Autodesk Inventor part; units mm, degrees
ref_plane "Work Plane1" through (0, 5, 0) normal (0, 1, 0) x (-1, 0, 0)
ref_plane "YZ Plane" through (0, 0, 0) normal (1, 0, 0) x (0, 1, 0)
ref_plane "XY Plane" through (0, 0, 0) normal (0, 0, 1) x (1, 0, 0)
sketch "Sketch5" plane through (0, 0, 0) normal (1, 0, 0) x (0, 1, 0)
  line L0 (0, 0) -> (5, 0)
  line L1 (5, 0) -> (5, -1.5)
  line L2 (5, -1.5) -> (3.55, -1.5)
  line L3 (3.55, -1.5) -> (3.55, -2.4)
  line L4 (3.55, -2.4) -> (5, -2.4)
  line L5 (5, -2.4) -> (5, -23.9)
  line L6 (5, -23.9) -> (3.55, -23.9)
  line L7 (3.55, -23.9) -> (3.55, -24.8)
  line L8 (3.55, -24.8) -> (5, -24.8)
  line L9 (5, -24.8) -> (5, -50)
  line L10 (5, -50) -> (0, -50)
  line L11 (0, -50) -> (0, 0)
  dimension "d14" = 0.9
  dimension "d15" = 1.5
  dimension "d16" = 0.9
  dimension "d17" = 50
  dimension "d18" = 10
  dimension "d19" = 7.1
  dimension "d28" = 23.3
revolve "Revolution2" add sketch "Sketch5" angle 360 about axis through (0, 0, -50) along (0, 0, 1)
ref_plane "Work Plane1" through (0, 5, 0) normal (0, 1, 0) x (-1, 0, 0)
sketch "Sketch6" plane through (0, 5, 0) normal (0, 1, 0) x (-1, 0, 0)
  line L0 (0, -5.5) -> (0, -9.5) construction
  line L1 (-2, -5.5) -> (-2, -9.5)
  line L2 (2, -9.5) -> (2, -5.5)
  arc A0 (2, -5.5) -> (-2, -5.5) centre (0, -5.5) ccw
  arc A1 (-2, -9.5) -> (2, -9.5) centre (0, -9.5) ccw
  line L3 (5, -1.5) -> (-5, -1.5)
  point P0 (0, 0)
  point P1 (0, -7.5)
  point P2 (0, -3.5)
  point P3 (0, -11.5)
  dimension "d22" = 4
  dimension "d23" = 8
  dimension "d24" = 2
extrude "Extrusion4" cut sketch "Sketch6" against normal blind 2.3
properties part number "gearbox_shaft2" material "Steel"
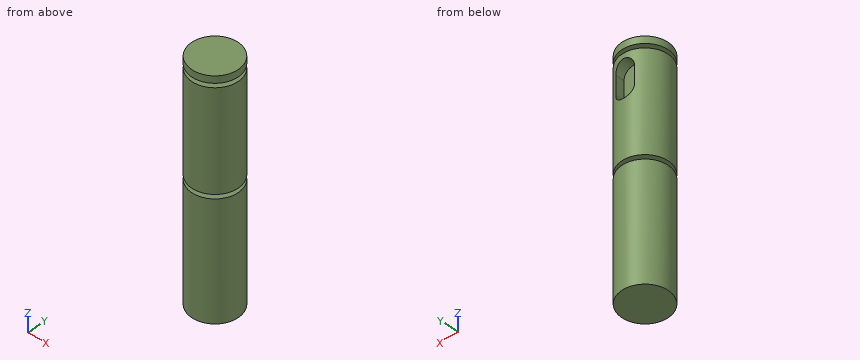
Can you work these out from the model? Positions are in its coordinate system, mm. Give positions to 0.01 mm unless a question says otherwise; leave off trailing zeros. Loops run counter-clockwise (first coordinate to the right, second up) from the corner with the lowest first, then second, coordinate; pieces in that order, holes last. Notation, with made-up numbers: M 51.25,64.25 L 90.25,64.25 A34 ccw 90.25,97.25 Z; hole C 77.25,-7.5 d6. An arc over 180 degrees is marked long. Use CSV: the item, a comma, the result in double quotes. Start each with the question number.
1. Imagine slicing it at A-A, the plane x = -4.25. Write out the boundary of the cut face in (y, z).
2. Imagine slicing it at D-D, the plane z = -41.5. Write out the boundary of the cut face in (x, y), plus the area to 3 significant figures.
3. If I drill on L1, parallel to Z at x = -1.75, y = -3.5; L2, parallel to Y at x = 3.75, z = -34.5; L3, parallel to Y at x = 1, z = -21, over which ranges is the centre line in solid material (lowest first)?
4. Imagine slicing it at B-B, the plane x = -0.5. Write out the boundary of the cut face in (y, z), plus the area to 3 significant figures.
5. Imagine slicing it at C-C, the plane y = -1.5. Write out the boundary of the cut face in (x, z), plus the area to 3 significant figures.
6. For P1, Ø4.5, axis at x = 0.5, z = -6, coming from the +Y side; P2, Ø1, axis at y = -3.5, z = -33, coming from the -X side; P3, Ø0.6, axis at y = 4, z = -8, coming from the +X side, each with a flat end and sliding along its axis, tell me the tip position at first contact or that it passes through.
Response values:
1,outline,"M -2.63,-50 L 2.63,-50 L 2.63,-24.8 L -2.63,-24.8 Z; M -2.63,-23.9 L 2.63,-23.9 L 2.63,-2.4 L -2.63,-2.4 Z; M -2.63,-1.5 L 2.63,-1.5 L 2.63,0 L -2.63,0 Z"
2,outline,"C 0,0 d10"
2,area,"78.5 mm^2"
3,L1,"-50 to -24.8, -23.9 to -2.4, -1.5 to 0"
3,L2,"-3.31 to 3.31"
3,L3,"-4.9 to 4.9"
4,outline,"M -4.97,-50 L 4.97,-50 L 4.97,-24.8 L 3.51,-24.8 L 3.51,-23.9 L 4.97,-23.9 L 4.97,-11.44 L 2.7,-11.44 L 2.7,-3.56 L 4.97,-3.56 L 4.97,-2.4 L 3.51,-2.4 L 3.51,-1.5 L 4.97,-1.5 L 4.97,0 L -4.97,0 L -4.97,-1.5 L -3.51,-1.5 L -3.51,-2.4 L -4.97,-2.4 L -4.97,-23.9 L -3.51,-23.9 L -3.51,-24.8 L -4.97,-24.8 Z"
4,area,"474 mm^2"
5,outline,"M -4.77,-50 L 4.77,-50 L 4.77,-24.8 L 3.22,-24.8 L 3.22,-23.9 L 4.77,-23.9 L 4.77,-2.4 L 3.22,-2.4 L 3.22,-1.5 L 4.77,-1.5 L 4.77,0 L -4.77,0 L -4.77,-1.5 L -3.22,-1.5 L -3.22,-2.4 L -4.77,-2.4 L -4.77,-23.9 L -3.22,-23.9 L -3.22,-24.8 L -4.77,-24.8 Z"
5,area,"471 mm^2"
6,P1,"y = 4.88"
6,P2,"x = -4"
6,P3,"x = 3.36"
